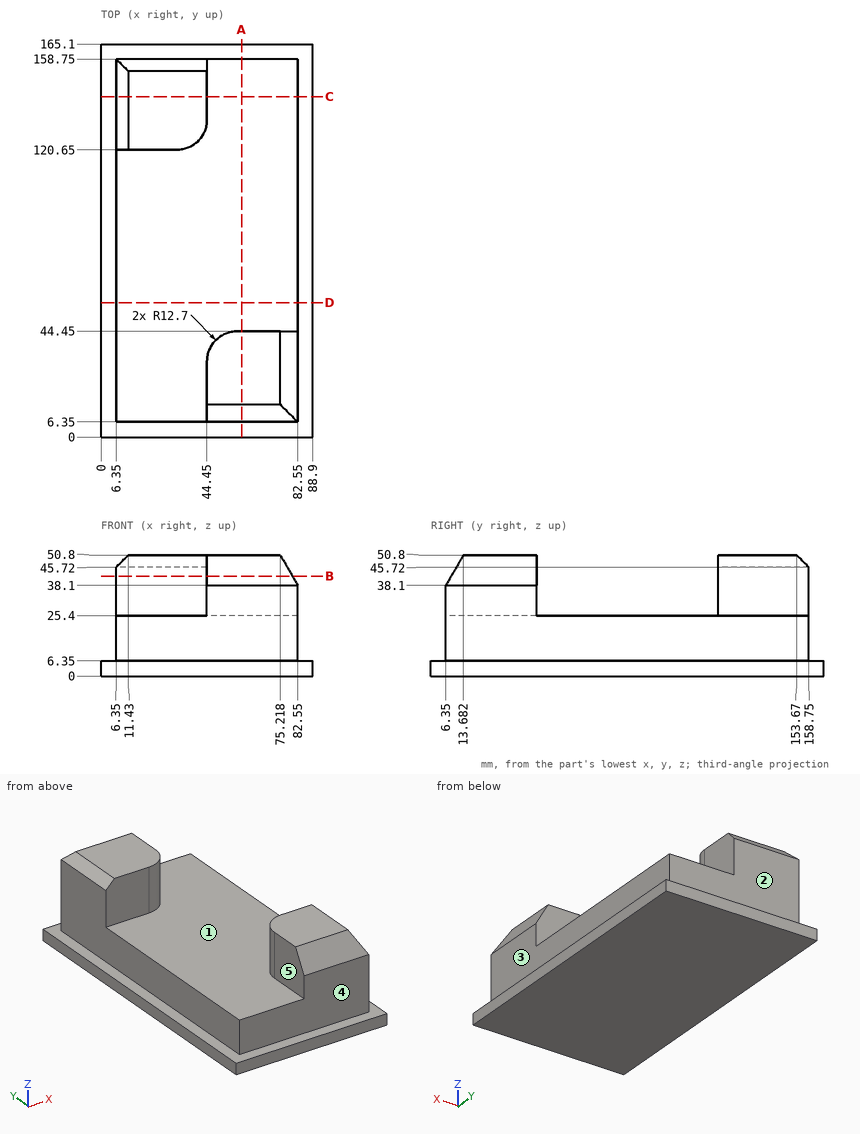
Print and shaded views of the part. All mm, measured from the part's lowest x, y and z. A direction names the side the tool comes from. Round coordinates to 2 decimals unless told otherwise and drop trailing zeros. Order: outer loops, then holes, each group sorted by start corner. A loop starts at its lowest first (then second) coordinate and runs counter-clockwise, first axis right, second up.
Q1. Slice it at D-D (y = 56.5). Write the cut outline in (x, z), and give its area (3 significant figures).
Q2. Wall check: L1, parallel to Y at x = 50, z = 18.5; L2, parallel to X at y = 72.5, z = 23; L3, parallel to Z at x = 37, y = 70. Give the ranges that are in metal, low to high.
Q3. Drop flat-ended pins along their axis: pin 1 (3 mm diameter, centred on x = 17.5, z = 11, fed in from -Y); pin 2 (10 mm diameter, centred on y = 137, z = 20, fed in from +X); pin 3 (12 mm diameter, centred on x = 40.5, z = 33.5, fed in from +Y); pin 4 (6 mm diameter, centred on y = 45.5, z = 7.5, fed in from +X). Give the stop position or say it passes through.
Q4. Slice it at C-C (y = 143). Write the cut outline in (x, z).
Q5. Which spindle directions (+Z, -Z, +X, -X, +Y, -Y) get a long thin tool onto all of the face, cutting with end or side? Do the marked faces 1, 2, 3, 4 and 5. Say none if no direction does.
Q6. Slice it at B-B (z = 42). Write the cut outline in (x, y), and give its area (3 significant figures).
Q7. Slice it at A-A (x = 59). Write the cut outline in (y, z).
Results below:
1. outline: (0, 0) - (88.9, 0) - (88.9, 6.35) - (82.55, 6.35) - (82.55, 25.4) - (6.35, 25.4) - (6.35, 6.35) - (0, 6.35) - close
1. area: 2,020 mm2
2. L1: y = 6.35 to 158.75
2. L2: x = 6.35 to 82.55
2. L3: z = 0 to 25.4
3. pin 1: stops at y = 6.35
3. pin 2: stops at x = 82.55
3. pin 3: stops at y = 158.75
3. pin 4: stops at x = 88.9
4. outline: (0, 0) - (88.9, 0) - (88.9, 6.35) - (82.55, 6.35) - (82.55, 25.4) - (44.45, 25.4) - (44.45, 50.8) - (11.43, 50.8) - (6.35, 45.72) - (6.35, 6.35) - (0, 6.35) - close
5. face 1: +Z
5. face 2: +Z, +X, -X, +Y
5. face 3: +Z, +X, +Y, -Y
5. face 4: +Z, +X, -X, -Y
5. face 5: +Z, -X, -Y
6. outline: (6.35, 120.65) - (31.75, 120.65) arc R12.7 ccw to (44.45, 133.35) - (44.45, 158.75) - (6.35, 158.75) - close; (44.45, 8.6) - (80.3, 8.6) - (80.3, 44.45) - (57.15, 44.45) arc R12.7 ccw to (44.45, 31.75) - close
6. area: 2,670 mm2
7. outline: (0, 0) - (165.1, 0) - (165.1, 6.35) - (158.75, 6.35) - (158.75, 25.4) - (44.45, 25.4) - (44.45, 50.8) - (13.68, 50.8) - (6.35, 38.1) - (6.35, 6.35) - (0, 6.35) - close
